Here's how the part is built. I have some questions about the finished solid (model axes, mm). Face numbers are marked on the shaded views. A direction names the side the tool comes from. Give positions to 0.01 mm unless a question says otherwise; leave off trailing zeros. Loops run counter-clockwise (first coordinate to the right, second up) from the corner with the lowest first, then second, coordinate; pieces in that order, holes last. Notation, with made-up numbers: (-22.75, 57.5) - (0.25, 57.5) arc R13 ccw to (0.25, 67.5) - close; hole circle Ø3 at (1, -4.75). An arc over 180 degrees is marked (long way). One line per item, written item: value. Start each with the question number.
```python
from build123d import *

# Parameters (mm, degrees)
BOSS_EXTRUDE1_DEPTH     = 18
SKETCH2_W               = 20
SKETCH2_H               = 8
BOSS_EXTRUDE2_DEPTH     = 2
CUT_EXTRUDE1_DEPTH      = 23.27666941
CUT_EXTRUDE1_DEPTH_BACK = 23.27666941
SKETCH3_W               = 9.3
SKETCH3_H               = 2
SKETCH4_R               = 1.4
BOSS_EXTRUDE3_DEPTH     = 2
FILLET1_R               = 0.5


with BuildPart() as part:
    # Sketch1 → Boss-Extrude1 (new body)
    with BuildSketch(Plane.XY):
        Polygon((-4.95, -3.4), (4.95, -3.4), (2.45, 0), (2.45, 0.5), (-2.45, 0.5), (-2.45, 0), align=None)
    extrude(amount=BOSS_EXTRUDE1_DEPTH)

    # Sketch2 → Boss-Extrude2 (add)
    with BuildSketch(Plane(origin=(0, 0, 0), x_dir=(-1, 0, 0), z_dir=(0, 0, -1))):
        with Locations((0, 4.5)):
            Rectangle(SKETCH2_W, SKETCH2_H)
    extrude(amount=-BOSS_EXTRUDE2_DEPTH)

    # Sketch3 → Cut-Extrude1 (cut, two sides: drawn at the far end of the back side and taken through both)
    with BuildSketch(Plane(origin=(0, 0, 0), x_dir=(0, 0, -1), z_dir=(1, 0, 0)).offset(-CUT_EXTRUDE1_DEPTH_BACK)):
        with Locations((-8.35, -2.4)):
            Rectangle(SKETCH3_W, SKETCH3_H)
    extrude(amount=CUT_EXTRUDE1_DEPTH + CUT_EXTRUDE1_DEPTH_BACK, mode=Mode.SUBTRACT)

    # Sketch4 → Boss-Extrude3 (add)
    with BuildSketch(Plane(origin=(0, 0, 0), x_dir=(-1, 0, 0), z_dir=(0, 0, -1))):
        with Locations((-6.2, 3)):
            Circle(SKETCH4_R)
        with Locations(Location((6.2, 3, 0), (0, 0, 180))):
            Circle(SKETCH4_R)
    extrude(amount=BOSS_EXTRUDE3_DEPTH)

    # Fillet1
    fillet1_edges = [part.edges().sort_by_distance(p)[0] for p in [
        (7.6, 3, -2),
        (-7.6, 3, -2),
    ]]
    fillet(fillet1_edges, radius=FILLET1_R)


solid = part.part
```
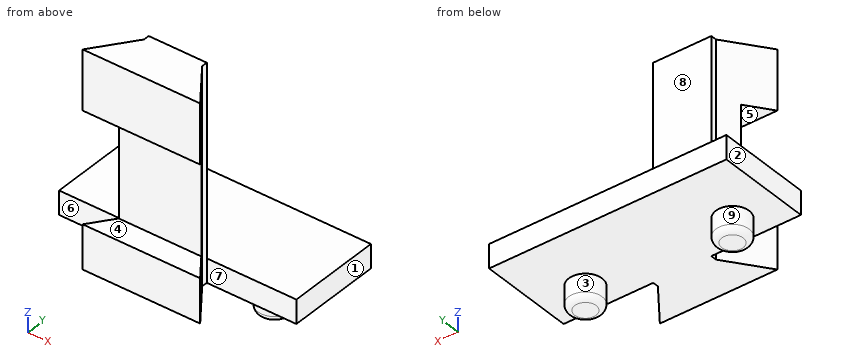
(1) If we section it at C-C on z = 13.75: List the corners of the cut face in (x, y) for me, plus the area to 3 significant figures.
(2) If we mould it in two halves opening along X, with no side actions, what happens to the marked faces 1, 2, 3 and 4? For each: pulls with the +X half, pulls with the -X half, needs draft (parallel to the pull), parting line crosses it, or undercut.
(3) If we section it at A-A on y = -1.75: List the corners of the cut face in (x, z) for me.
(4) If we section it at D-D on y = 3: List the corners of the cut face in (x, z) for me, plus the area to 3 significant figures.
(5) If we section it at B-B on x = -6.2: List the corners of the cut face in (y, z) for me.
(6) For the marked faces 5, 6, 7, 8 and 9, which set-ups out of +Z, -Z, +X, -X, +Y, -Y let a thin tool reach every point of the face, with its end or its side?
(7) Please list where these lines run through material, in increasing order: probe 1 along Z at (x, y) = (3.75, -2.5); probe 2 along Z at (x, y) = (-1.25, -0.5); probe 3 along Z at (x, y) = (-3.25, 3.75). Write a range as from..to.
(8) Will these pins go through, and if not, where does the flat tip stop? pin 1 (6 mm diameter, centred on x = 0.5, y = 3.5, fed in from -Z); pin 2 (6 mm diameter, centred on x = 3.5, z = 9, fed in from +Y); pin 3 (1.6 mm diameter, centred on x = -6, z = 1.5, fed in from -Y).
Found:
1. outline: (-4.95, -3.4) - (4.95, -3.4) - (2.45, 0) - (2.45, 0.5) - (-2.45, 0.5) - (-2.45, 0) - close
1. area: 27.6 mm^2
2. face 1: pulls with the +X half
2. face 2: pulls with the -X half
2. face 3: undercut
2. face 4: needs draft
3. outline: (-3.74, 0) - (3.74, 0) - (3.74, 3.7) - (-3.74, 3.7) - close; (-3.74, 13) - (3.74, 13) - (3.74, 18) - (-3.74, 18) - close
4. outline: (-10, 0) - (-7.6, 0) - (-7.6, -1.5) arc R0.5 ccw to (-7.1, -2) - (-5.3, -2) arc R0.5 ccw to (-4.8, -1.5) - (-4.8, 0) - (4.8, 0) - (4.8, -1.5) arc R0.5 ccw to (5.3, -2) - (7.1, -2) arc R0.5 ccw to (7.6, -1.5) - (7.6, 0) - (10, 0) - (10, 2) - (-10, 2) - close
4. area: 51.0 mm^2
5. outline: (0.5, 0) - (1.6, 0) - (1.6, -1.5) arc R0.5 ccw to (2.1, -2) - (3.9, -2) arc R0.5 ccw to (4.4, -1.5) - (4.4, 0) - (8.5, 0) - (8.5, 2) - (0.5, 2) - close
6. face 5: +X, -X, -Y
6. face 6: +Z, -Z, -X
6. face 7: +Z, -Z, +X
6. face 8: +Z, +X, -X, +Y
6. face 9: -Z
7. probe 1: 0..3.7, 13..18
7. probe 2: 0..18
7. probe 3: 0..2
8. pin 1: z = 0
8. pin 2: y = 0.5
8. pin 3: y = 0.5
